Could you check a few things on this model? Use its own coordinates, in mm. A direction names the side the tool comes from. Coordinates: 2 decimals unless noted, no trailing zeros. Loops run counter-clockwise (first coordinate to the right, second up) from the corner with the lowest first, then second, coordinate; pieces in that order, holes last. Notation, with made-up numbers: (42.25, -38.5) - (74.25, -38.5) arc R31 cw to (74.25, -12.5) - close; hole circle Ø11 at (85, -22.75). An arc over 180 degrees is marked (long way). Put each result on its own line as item: value. Start each with the question number.
```python
from build123d import *

# Parameters (mm, degrees)
F2_W     = 22.352
F2_H     = 63.5
F3_DEPTH = 66.548
F0_W     = 172.72
F0_H     = 22.352
F4_DEPTH = 66.548
F1_W     = 22.352
F1_H     = 41.148
F5_DEPTH = 66.548


with BuildPart() as f3:
    # F2 (on Right) → F3 (new body)
    with BuildSketch(Plane.YZ):
        with Locations((-74.962673, 20.931003)):
            Rectangle(F2_W, F2_H)
    extrude(amount=-F3_DEPTH)

    # F0 (on Right) → F4 (join)
    with BuildSketch(Plane.YZ):
        Rectangle(F0_W, F0_H)
    extrude(amount=-F4_DEPTH)

    # F1 (on Right) → F5 (join)
    with BuildSketch(Plane.YZ):
        with Locations((75.032448, -9.758694)):
            Rectangle(F1_W, F1_H)
    extrude(amount=-F5_DEPTH)


solid = f3.part
```
(1) I want a section at B-B on z = 38. List the corners of the cut face in (x, y) for me.
(2) I want a section at C-C on y = 28. List the corners of the cut face in (x, z) for me, and give its area (3 significant figures).
(3) For pin 1 Ø20 at (x, y) = (-38.5, -12) entering from +Z; pin 2 Ø5.5 at (x, z) = (-44.5, -24) entering from +Y; pin 3 Ø12 at (x, y) = (-50, -56.5) entering from -Z, each with a flat end and sliding along its axis, tell me the tip position at first contact or that it passes through.
(4) Which directions (+Z, -Z, +X, -X, +Y, -Y) give clear straight access to the entire face, cutting with the end or side of a thin tool? Please do faces 1 (the flat face through (-33, -12, -11.176)), 2 (the flat face through (-33, 86.208, -21)), 3 (the flat face through (-33, 10, 11.176)).
(5) I want a section at A-A on x = -45.5. List the corners of the cut face in (y, z) for me, and give its area (3 significant figures).
(6) I need wall thicknesses on L1, parallel to Y at x = -23, z = 38; L2, parallel to Z at x = -3.5, y = 44; L3, parallel to Y at x = -21, z = -24. Which ranges of each line are inside material? Lowest first, please. Write a range as [from, to].
Answer sheet:
1. outline: (-66.55, -86.14) - (0, -86.14) - (0, -63.79) - (-66.55, -63.79) - close
2. outline: (-66.55, -11.18) - (0, -11.18) - (0, 11.18) - (-66.55, 11.18) - close
2. area: 1,490 mm^2
3. pin 1: stops at z = 11.18
3. pin 2: stops at y = 86.21
3. pin 3: stops at z = -11.18
4. face 1: -Z, +X, -X, -Y
4. face 2: -Z, +X, -X, +Y
4. face 3: +Z, +X, -X, +Y
5. outline: (-86.36, -11.18) - (63.86, -11.18) - (63.86, -30.33) - (86.21, -30.33) - (86.21, -11.18) - (86.36, -11.18) - (86.36, 11.18) - (-63.79, 11.18) - (-63.79, 52.68) - (-86.14, 52.68) - (-86.14, 11.18) - (-86.36, 11.18) - close
5. area: 5,220 mm^2
6. L1: y = [-86.14, -63.79]
6. L2: z = [-11.18, 11.18]
6. L3: y = [63.86, 86.21]
